The model under review builds one solid part; all positions refer to its coordinate system, in mm. Face numbers are marked on the shaded views. A direction names the side the tool comes from. Give positions to 0.01 mm unless a question says otherwise; leave off trailing zeros. Order: outer loops, then holes, each group sorted by start corner. A loop starts at its lowest first (then second) coordinate and runs counter-clockwise, first axis right, second up. Notation, with made-up numbers: (-2.5, -29) - (11.5, -29) arc R14 cw to (11.5, -17) - close; hole circle Ø2 at (-16, 65). An arc over 180 degrees is marked (long way). Write item = value, one per line. Start each with the question number.
1. Mouldability with a two-part tool opening along Y and no side actions: class the marked faces 3, 4, 5 and 6 as pulls with the +Y half, pulls with the -Y half, needs draft (parallel to the pull), parting line crosses it, or undercut.
2. We need section D-D, the plane y = -1. Give the boundary of the cut face in (x, z).
3. Wall thickness on probe 1 along Y at (x, z) = (17, 9.25); probe 2 along X at (y, z) = (-13.25, 10.5): over which ranges is each line inside the solid? List them lowest first.
4. We need section C-C, the plane z = 7.75. Give the boundary of the cut face in (x, y).
5. We need section B-B, the plane y = -10. Give the boundary of the cut face in (x, z), and give its area (3 significant figures).
6. We need section A-A, the plane x = 30.5. Give the boundary of the cut face in (y, z), and give its area (3 significant figures).
7. Machinability: for the marked faces 1 and 2, which of the approach directions +Z, -Z, +X, -X, +Y, -Y give a long, thin tool a straight path to every point of the face, cutting with its end or side? Answer none if there is none.
8. For P1, Ø5.5, axis at x = 14.5, z = 12, coming from the +Y side; P2, Ø2, axis at x = 32.5, y = -5, coming from the +Z side; P3, Ø10, axis at y = -9.5, z = 16.5, coming from the +X side; P4, Ø2, axis at x = 22.5, z = 12.5, coming from the +Y side, all flat-tipped, find the tip position at first contact; note any pin that passes through.
from build123d import *

# Parameters (mm, degrees)
CYLINDER002_R             = 3
CYLINDER002_DEPTH         = 2
BOX001_W                  = 8
BOX001_H                  = 6
BOX001_DEPTH              = 2
CYLINDER003_R             = 3
CYLINDER003_DEPTH         = 2
FUSION001_PLACEMENT_ANGLE = 270
CYLINDER_R                = 2
CYLINDER_DEPTH            = 2
BOX_W                     = 30
BOX_H                     = 4
BOX_DEPTH                 = 2
CYLINDER001_R             = 2
CYLINDER001_DEPTH         = 2
PAD001_DEPTH              = 16
PAD_DEPTH                 = 20


with BuildPart() as cylinder002:
    # Cylinder002 → Cylinder002 (new body)
    with BuildSketch(Plane.XY):
        Circle(CYLINDER002_R)
    extrude(amount=CYLINDER002_DEPTH)


with BuildPart() as cube001:
    # Box001 → Box001 (new body)
    with BuildSketch(Plane(origin=(0, -3, 0), x_dir=(1, 0, 0), z_dir=(0, 0, 1))):
        with Locations((4, 3)):
            Rectangle(BOX001_W, BOX001_H)
    extrude(amount=BOX001_DEPTH)


with BuildPart() as longhole002:
    # Cylinder003 → Cylinder003 (new body)
    with BuildSketch(Plane(origin=(8, 0, 0), x_dir=(1, 0, 0), z_dir=(0, 0, 1))):
        Circle(CYLINDER003_R)
    extrude(amount=CYLINDER003_DEPTH)

    # Fusion001: union Cylinder002, Cube001
    add(cylinder002.part)
    add(cube001.part)


with BuildPart() as longhole002_1:
    # Fusion001 placement: moved
    add(longhole002.part.moved(Location((2, -10, 7))).rotate(Axis((2, -10, 7), (0, 1, 0)), FUSION001_PLACEMENT_ANGLE))


with BuildPart() as cylinder:
    # Cylinder → Cylinder (new body)
    with BuildSketch(Plane.XY):
        Circle(CYLINDER_R)
    extrude(amount=CYLINDER_DEPTH)


with BuildPart() as cube:
    # Box → Box (new body)
    with BuildSketch(Plane(origin=(0, -2, 0), x_dir=(1, 0, 0), z_dir=(0, 0, 1))):
        with Locations((15, 2)):
            Rectangle(BOX_W, BOX_H)
    extrude(amount=BOX_DEPTH)


with BuildPart() as longhole1:
    # Cylinder001 → Cylinder001 (new body)
    with BuildSketch(Plane(origin=(30, 0, 0), x_dir=(1, 0, 0), z_dir=(0, 0, 1))):
        Circle(CYLINDER001_R)
    extrude(amount=CYLINDER001_DEPTH)

    # Fusion: union Cylinder, Cube
    add(cylinder.part)
    add(cube.part)


with BuildPart() as longhole1_1:
    # Fusion placement: moved
    add(longhole1.part.moved(Location((6, -10, 0))))


with BuildPart() as body001:
    # Sketch001 → Pad001 (new body)
    with BuildSketch(Plane.XZ):
        Polygon((2, 20), (40, 2), (2, 2), align=None)
    extrude(amount=PAD001_DEPTH)


with BuildPart() as body001_1:
    # Body001 placement: moved
    add(body001.part.moved(Location((0, -2, 0))))


with BuildPart() as modularmountingbracket:
    # Sketch → Pad (new body)
    with BuildSketch(Plane.XZ):
        Polygon((0, 20), (0, 0), (40, 0), (40, 2), (2, 20), align=None)
    extrude(amount=PAD_DEPTH)

    # Cut: cut Body001
    add(body001_1.part, mode=Mode.SUBTRACT)

    # Cut001: cut LongHole1
    add(longhole1_1.part, mode=Mode.SUBTRACT)

    # Cut002: cut LongHole002
    add(longhole002_1.part, mode=Mode.SUBTRACT)


solid = modularmountingbracket.part
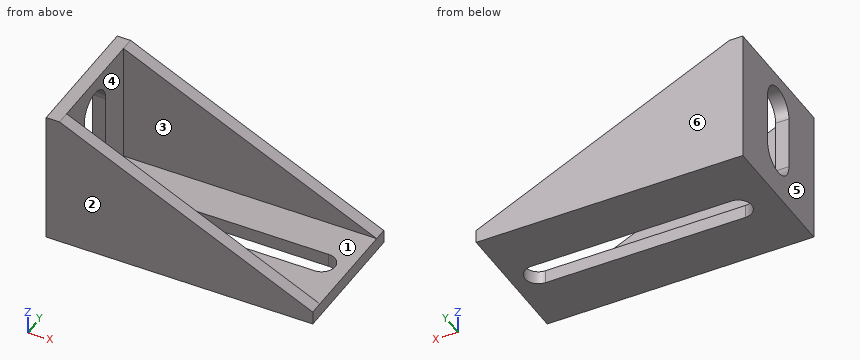
Model answer:
q1.face_3 = undercut
q1.face_4 = undercut
q1.face_5 = needs draft
q1.face_6 = pulls with the +Y half
q2.outline = (0, 0) - (40, 0) - (40, 2) - (2, 20) - (0, 20) - close
q3.probe_1 = -20 to -18, -2 to 0
q3.probe_2 = 0 to 2
q4.outline = (0, -20) - (27.86, -20) - (27.86, -18) - (2, -18) - (2, -13) - (0, -13) - close; (0, -7) - (2, -7) - (2, -2) - (27.86, -2) - (27.86, 0) - (0, 0) - close
q5.outline = (0, 0) - (4, 0) - (4, 2) - (2, 2) - (2, 4) - (0, 4) - close; (0, 18) - (2, 18) - (2, 20) - (0, 20) - close; (38, 0) - (40, 0) - (40, 2) - (38, 2) - close
q5.area = 20.0 mm2
q6.outline = (-20, 0) - (-12, 0) - (-12, 2) - (-18, 2) - (-18, 6.5) - (-20, 6.5) - close; (-8, 0) - (0, 0) - (0, 6.5) - (-2, 6.5) - (-2, 2) - (-8, 2) - close
q6.area = 50.0 mm2
q7.face_1 = +Z, +X
q7.face_2 = +Z, -Z, +X, -X, -Y
q8.P1 = 0
q8.P2 = 2
q8.P3 = 2
q8.P4 = through
